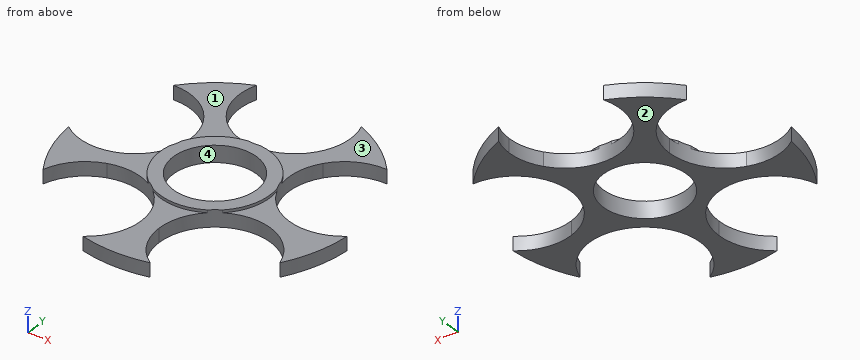
from build123d import *

# Parameters (mm, degrees)
F0_R     = 60
F1_DEPTH = 5
F2_R     = 19.75
F3_DEPTH = 1
F4_DEPTH = 25
F5_R     = 60
F6_DEPTH = 25
F7_R     = 15
F8_DEPTH = 25


with BuildPart() as f1:
    # F0 (on Top) → F1 (new body)
    with BuildSketch(Plane.XY):
        Circle(F0_R)
        with BuildLine():
            ThreePointArc((57.5667323937, 12.2061712778), (49.3224374395, -3.9741686097), (31.3863925062, -6.8149590481))
            Line((31.3863925062, -6.8149590481), (29.3978573531, -12.9350409519))
            ThreePointArc((29.3978573531, -12.9350409519), (39.3978573531, -20.200466232), (43.2175174656, -31.9561712778))
            ThreePointArc((43.2175174656, -31.9561712778), (23.2175174656, -51.9561712778), (3.2175174656, -31.9561712778))
            Line((3.2175174656, -31.9561712778), (-3.2175174656, -31.9561712778))
            ThreePointArc((-3.2175174656, -31.9561712778), (-34.9732225114, -48.1365111653), (-29.3978573531, -12.9350409519))
            Line((-29.3978573531, -12.9350409519), (-31.3863925062, -6.8149590481))
            ThreePointArc((-31.3863925062, -6.8149590481), (-56.5878627196, 18.3865111653), (-21.3863925062, 23.9618763237))
            Line((-21.3863925062, 23.9618763237), (-16.1803398875, 27.7442949542))
            ThreePointArc((-16.1803398875, 27.7442949542), (-6.1803398875, 58.5211303259), (20, 39.5))
            ThreePointArc((20, 39.5), (19.0211303259, 33.3196601125), (16.1803398875, 27.7442949542))
            Line((16.1803398875, 27.7442949542), (21.3863925062, 23.9618763237))
            ThreePointArc((21.3863925062, 23.9618763237), (43.7470722812, 31.2273016037), (57.5667323937, 12.2061712778))
        make_face(mode=Mode.SUBTRACT)
        with BuildLine():
            Line((-37.5667323937, 12.2061712778), (-21.3863925062, 23.9618763237))
            ThreePointArc((-21.3863925062, 23.9618763237), (-56.5878627196, 18.3865111653), (-31.3863925062, -6.8149590481))
            Line((-31.3863925062, -6.8149590481), (-37.5667323937, 12.2061712778))
        make_face()
        with BuildLine():
            ThreePointArc((-17.5667323937, 12.2061712778), (-18.5456020678, 18.3865111653), (-21.3863925062, 23.9618763237))
            Line((-21.3863925062, 23.9618763237), (-37.5667323937, 12.2061712778))
            Line((-37.5667323937, 12.2061712778), (-31.3863925062, -6.8149590481))
            ThreePointArc((-31.3863925062, -6.8149590481), (-21.3863925062, 0.450466232), (-17.5667323937, 12.2061712778))
        make_face()
        with BuildLine():
            ThreePointArc((-29.3978573531, -12.9350409519), (-34.9732225114, -48.1365111653), (-3.2175174656, -31.9561712778))
            Line((-3.2175174656, -31.9561712778), (-23.2175174656, -31.9561712778))
            Line((-23.2175174656, -31.9561712778), (-29.3978573531, -12.9350409519))
        make_face()
        with BuildLine():
            Line((-23.2175174656, -31.9561712778), (-3.2175174656, -31.9561712778))
            ThreePointArc((-3.2175174656, -31.9561712778), (-11.4618124197, -15.7758313903), (-29.3978573531, -12.9350409519))
            Line((-29.3978573531, -12.9350409519), (-23.2175174656, -31.9561712778))
        make_face()
        with BuildLine():
            ThreePointArc((43.2175174656, -31.9561712778), (39.3978573531, -20.200466232), (29.3978573531, -12.9350409519))
            Line((29.3978573531, -12.9350409519), (23.2175174656, -31.9561712778))
            Line((23.2175174656, -31.9561712778), (3.2175174656, -31.9561712778))
            ThreePointArc((3.2175174656, -31.9561712778), (23.2175174656, -51.9561712778), (43.2175174656, -31.9561712778))
        make_face()
        with BuildLine():
            Line((23.2175174656, -31.9561712778), (29.3978573531, -12.9350409519))
            ThreePointArc((29.3978573531, -12.9350409519), (11.4618124197, -15.7758313903), (3.2175174656, -31.9561712778))
            Line((3.2175174656, -31.9561712778), (23.2175174656, -31.9561712778))
        make_face()
        with BuildLine():
            Line((29.3978573531, -12.9350409519), (31.3863925062, -6.8149590481))
            ThreePointArc((31.3863925062, -6.8149590481), (18.5456020678, 6.0258313903), (21.3863925062, 23.9618763237))
            Line((21.3863925062, 23.9618763237), (16.1803398875, 27.7442949542))
            ThreePointArc((16.1803398875, 27.7442949542), (0, 19.5), (-16.1803398875, 27.7442949542))
            Line((-16.1803398875, 27.7442949542), (-21.3863925062, 23.9618763237))
            ThreePointArc((-21.3863925062, 23.9618763237), (-18.5456020678, 18.3865111653), (-17.5667323937, 12.2061712778))
            ThreePointArc((-17.5667323937, 12.2061712778), (-21.3863925062, 0.450466232), (-31.3863925062, -6.8149590481))
            Line((-31.3863925062, -6.8149590481), (-29.3978573531, -12.9350409519))
            ThreePointArc((-29.3978573531, -12.9350409519), (-11.4618124197, -15.7758313903), (-3.2175174656, -31.9561712778))
            Line((-3.2175174656, -31.9561712778), (3.2175174656, -31.9561712778))
            ThreePointArc((3.2175174656, -31.9561712778), (11.4618124197, -15.7758313903), (29.3978573531, -12.9350409519))
        make_face()
        with BuildLine():
            Line((31.3863925062, -6.8149590481), (37.5667323937, 12.2061712778))
            Line((37.5667323937, 12.2061712778), (21.3863925062, 23.9618763237))
            ThreePointArc((21.3863925062, 23.9618763237), (18.5456020678, 6.0258313903), (31.3863925062, -6.8149590481))
        make_face()
        with BuildLine():
            Line((21.3863925062, 23.9618763237), (37.5667323937, 12.2061712778))
            Line((37.5667323937, 12.2061712778), (31.3863925062, -6.8149590481))
            ThreePointArc((31.3863925062, -6.8149590481), (49.3224374395, -3.9741686097), (57.5667323937, 12.2061712778))
            ThreePointArc((57.5667323937, 12.2061712778), (43.7470722812, 31.2273016037), (21.3863925062, 23.9618763237))
        make_face()
        with BuildLine():
            ThreePointArc((-16.1803398875, 27.7442949542), (0, 19.5), (16.1803398875, 27.7442949542))
            Line((16.1803398875, 27.7442949542), (0, 39.5))
            Line((0, 39.5), (-16.1803398875, 27.7442949542))
        make_face()
        with BuildLine():
            Line((0, 39.5), (16.1803398875, 27.7442949542))
            ThreePointArc((16.1803398875, 27.7442949542), (19.0211303259, 33.3196601125), (20, 39.5))
            ThreePointArc((20, 39.5), (-6.1803398875, 58.5211303259), (-16.1803398875, 27.7442949542))
            Line((-16.1803398875, 27.7442949542), (0, 39.5))
        make_face()
    extrude(amount=F1_DEPTH)

    # F2 (on face) → F3 (join)
    with BuildSketch(Plane.XY.offset(5)):
        Circle(F2_R)
    extrude(amount=F3_DEPTH)

    # F0 (on Top) → F4 (cut)
    with BuildSketch(Plane.XY):
        with BuildLine():
            ThreePointArc((-29.3978573531, -12.9350409519), (-34.9732225114, -48.1365111653), (-3.2175174656, -31.9561712778))
            Line((-3.2175174656, -31.9561712778), (-23.2175174656, -31.9561712778))
            Line((-23.2175174656, -31.9561712778), (-29.3978573531, -12.9350409519))
        make_face()
        with BuildLine():
            Line((-23.2175174656, -31.9561712778), (-3.2175174656, -31.9561712778))
            ThreePointArc((-3.2175174656, -31.9561712778), (-11.4618124197, -15.7758313903), (-29.3978573531, -12.9350409519))
            Line((-29.3978573531, -12.9350409519), (-23.2175174656, -31.9561712778))
        make_face()
        with BuildLine():
            ThreePointArc((43.2175174656, -31.9561712778), (39.3978573531, -20.200466232), (29.3978573531, -12.9350409519))
            Line((29.3978573531, -12.9350409519), (23.2175174656, -31.9561712778))
            Line((23.2175174656, -31.9561712778), (3.2175174656, -31.9561712778))
            ThreePointArc((3.2175174656, -31.9561712778), (23.2175174656, -51.9561712778), (43.2175174656, -31.9561712778))
        make_face()
        with BuildLine():
            Line((23.2175174656, -31.9561712778), (29.3978573531, -12.9350409519))
            ThreePointArc((29.3978573531, -12.9350409519), (11.4618124197, -15.7758313903), (3.2175174656, -31.9561712778))
            Line((3.2175174656, -31.9561712778), (23.2175174656, -31.9561712778))
        make_face()
        with BuildLine():
            Line((21.3863925062, 23.9618763237), (37.5667323937, 12.2061712778))
            Line((37.5667323937, 12.2061712778), (31.3863925062, -6.8149590481))
            ThreePointArc((31.3863925062, -6.8149590481), (49.3224374395, -3.9741686097), (57.5667323937, 12.2061712778))
            ThreePointArc((57.5667323937, 12.2061712778), (43.7470722812, 31.2273016037), (21.3863925062, 23.9618763237))
        make_face()
        with BuildLine():
            Line((31.3863925062, -6.8149590481), (37.5667323937, 12.2061712778))
            Line((37.5667323937, 12.2061712778), (21.3863925062, 23.9618763237))
            ThreePointArc((21.3863925062, 23.9618763237), (18.5456020678, 6.0258313903), (31.3863925062, -6.8149590481))
        make_face()
        with BuildLine():
            ThreePointArc((-16.1803398875, 27.7442949542), (0, 19.5), (16.1803398875, 27.7442949542))
            Line((16.1803398875, 27.7442949542), (0, 39.5))
            Line((0, 39.5), (-16.1803398875, 27.7442949542))
        make_face()
        with BuildLine():
            Line((0, 39.5), (16.1803398875, 27.7442949542))
            ThreePointArc((16.1803398875, 27.7442949542), (19.0211303259, 33.3196601125), (20, 39.5))
            ThreePointArc((20, 39.5), (-6.1803398875, 58.5211303259), (-16.1803398875, 27.7442949542))
            Line((-16.1803398875, 27.7442949542), (0, 39.5))
        make_face()
        with BuildLine():
            Line((-37.5667323937, 12.2061712778), (-21.3863925062, 23.9618763237))
            ThreePointArc((-21.3863925062, 23.9618763237), (-56.5878627196, 18.3865111653), (-31.3863925062, -6.8149590481))
            Line((-31.3863925062, -6.8149590481), (-37.5667323937, 12.2061712778))
        make_face()
        with BuildLine():
            ThreePointArc((-17.5667323937, 12.2061712778), (-18.5456020678, 18.3865111653), (-21.3863925062, 23.9618763237))
            Line((-21.3863925062, 23.9618763237), (-37.5667323937, 12.2061712778))
            Line((-37.5667323937, 12.2061712778), (-31.3863925062, -6.8149590481))
            ThreePointArc((-31.3863925062, -6.8149590481), (-21.3863925062, 0.450466232), (-17.5667323937, 12.2061712778))
        make_face()
    extrude(amount=F4_DEPTH, mode=Mode.SUBTRACT)

    # F5 (on face) → F6 (cut)
    with BuildSketch(Plane.XY):
        Circle(F5_R)
        with BuildLine():
            ThreePointArc((18.7968074618, 46.332278481), (29.3892626146, 40.4508497187), (38.2560824185, 32.1942876609))
            ThreePointArc((38.2560824185, 32.1942876609), (51.9505253652, 26.1024477486), (57.5667323937, 12.2061712778))
            ThreePointArc((57.5667323937, 12.2061712778), (55.5407180163, 3.4348634598), (49.8731483099, -3.5593647834))
            ThreePointArc((49.8731483099, -3.5593647834), (47.5528258148, -15.4508497187), (42.4403666729, -26.435114463))
            ThreePointArc((42.4403666729, -26.435114463), (43.0222767944, -29.1684288351), (43.2175174656, -31.9561712778))
            ThreePointArc((43.2175174656, -31.9561712778), (32.6031319122, -49.6171520393), (12.0264933196, -48.5320868955))
            ThreePointArc((12.0264933196, -48.5320868955), (0, -50), (-12.0264933196, -48.5320868955))
            ThreePointArc((-12.0264933196, -48.5320868955), (-34.9732225114, -48.1365111653), (-42.4403666729, -26.435114463))
            ThreePointArc((-42.4403666729, -26.435114463), (-47.5528258148, -15.4508497187), (-49.8731483099, -3.5593647834))
            ThreePointArc((-49.8731483099, -3.5593647834), (-56.5878627196, 18.3865111653), (-38.2560824185, 32.1942876609))
            ThreePointArc((-38.2560824185, 32.1942876609), (-29.3892626146, 40.4508497187), (-18.7968074618, 46.332278481))
            ThreePointArc((-18.7968074619, 46.332278481), (0, 59.5), (18.7968074619, 46.332278481))
        make_face(mode=Mode.SUBTRACT)
    extrude(amount=F6_DEPTH, mode=Mode.SUBTRACT)

    # F7 (on face) → F8 (cut)
    with BuildSketch(Plane.XY.offset(6)):
        Circle(F7_R)
    extrude(amount=-F8_DEPTH, mode=Mode.SUBTRACT)


solid = f1.part
Verification items for the finished model (mm, model axes). Face numbers are marked on the shaded views. A direction names the side the tool comes from. Give positions to 0.01 mm unless a question says otherwise; leave off trailing zeros. Write each loop counter-clockwise with the first axis right and the second up, starting at its lowest first coordinate (ties: lowest second). Pieces come first, ordered by that corner, then holes.
(1) Mould release check, pull along X, two halves, no side actions. Record for the marked faces 3 and 4: +X half, -X half, draft (parallel to the pull), parting line (faces both ways), or undercut.
(2) Access from +Z, -Z, +X, -X, +Y, -Y to the whole of each face (thin tool, end or side, straight path). Record for the marked faces 1 and 2.
(3) Cross-section at D-D (y = 0). Enter the section's corners in (x, z).
(4) Cross-section at C-C (y = 38). Enter the section's corners in (x, z).
(5) Cross-section at B-B (z = 4). Enter the section's corners in (x, y).
(6) Cross-section at A-A (x = 0). Enter the section's corners in (y, z), plus the area to 3 significant figures.
(7) Gauge pin test, flat ends, axial feed: pin 1 (1.5 mm diameter, centred on y = 26, z = 4, fed in from +X); pin 2 (7 mm diameter, centred on x = -4.5, y = -28, fed in from +Z); pin 3 (3 mm diameter, centred on x = -13, z = 2, fed in from -Y). Record the tip position at first contact, or that the pin passes through.
(8) Material ranges on line 1 (Y direction, x = 0, z = 4.35); line 2 (X direction, y = -16.5, z = 1.7); line 3 (Y direction, x = 6, z = 2), recorded low to high.
Worked out:
1. face 3: draft
1. face 4: undercut
2. face 1: +Z, -X, +Y
2. face 2: -Z, +X, -X, +Y, -Y
3. outline: (-21.72, 0) - (-15, 0) - (-15, 6) - (-19.75, 6) - (-19.75, 5) - (-21.72, 5) - close; (15, 0) - (21.72, 0) - (21.72, 5) - (19.75, 5) - (19.75, 6) - (15, 6) - close
4. outline: (-32.5, 0) - (-19.94, 0) - (-19.94, 5) - (-32.5, 5) - close; (19.94, 0) - (32.5, 0) - (32.5, 5) - (19.94, 5) - close
5. outline: (-49.87, -3.56) arc R50 ccw to (-42.44, -26.44) arc R20 cw (long way) to (-12.03, -48.53) arc R50 ccw to (12.03, -48.53) arc R20 cw (long way) to (42.44, -26.44) arc R50 ccw to (49.87, -3.56) arc R20 cw (long way) to (38.26, 32.19) arc R50 ccw to (18.8, 46.33) arc R20 cw (long way) to (-18.8, 46.33) arc R50 ccw to (-38.26, 32.19) arc R20 cw (long way) to start; hole circle Ø30 at (0, 0)
6. outline: (-50, 0) - (-15, 0) - (-15, 6) - (-19.75, 6) - (-19.75, 5) - (-50, 5) - close; (15, 0) - (19.5, 0) - (19.5, 6) - (15, 6) - close
6. area: 207 mm2
7. pin 1: stops at x = 23.84
7. pin 2: stops at z = 5
7. pin 3: stops at y = -48.66
8. line 1: y = -50 to -15, 15 to 19.5
8. line 2: x = -47.2 to -35.91, -10.52 to 10.52, 35.91 to 47.2
8. line 3: y = -49.64 to -42.13, -21.78 to -13.75, 13.75 to 20.42
